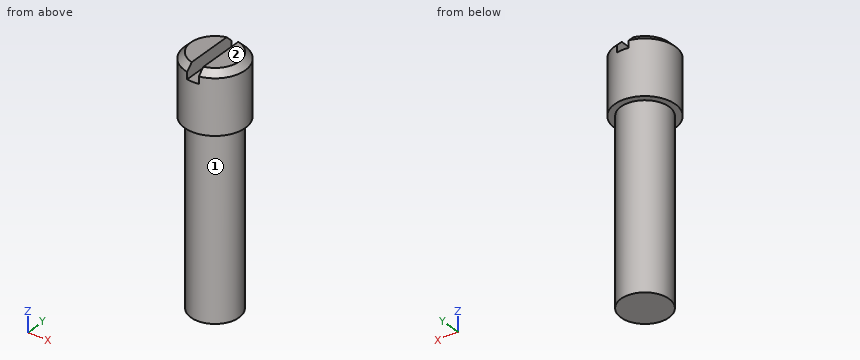
from build123d import *

# Parameters (mm, degrees)
ESQUISSE3_W             = 3
ESQUISSE3_H             = 24
CHANFREIN1_SIZE         = 0.6
ESQUISSE6_R             = 3.5
ENL_V_MAT_EXTRU_1_DEPTH = 25.50510151
ESQUISSE7_OUTSIDE_W     = 13.092
ESQUISSE7_OUTSIDE_H     = 13.092
ESQUISSE7_OUTSIDE_R     = 2.375
ENL_V_MAT_EXTRU_2_DEPTH = 18
ESQUISSE8_W             = 1.15
ESQUISSE8_H             = 7.450711795
ENL_V_MAT_EXTRU_3_DEPTH = 1.3


with BuildPart() as part:
    # Esquisse1 → Base-R_volution (revolve)
    with BuildSketch(Plane(origin=(0, 0, 0), x_dir=(1, 0, 0), z_dir=(0, 1, 0)), mode=Mode.PRIVATE) as base_r_volution_sk:
        with BuildLine():
            Line((0, 0), (3.5, 0))
            Line((3.5, 0), (3.5, 3.6))
            ThreePointArc((3.5, 3.6), (3.382842712, 3.882842712), (3.1, 4))
            Line((3.1, 4), (0, 4))
            Line((0, 4), (0, 0))
        make_face()
    revolve(base_r_volution_sk.sketch.rotate(Axis((0, 0, 0), (0, 0, -1)), 180), axis=Axis((0, 0, 0), (0, 0, -1)))

    # Esquisse3 → Boss.-R_vol.1 (revolve)
    with BuildSketch(Plane(origin=(0, 0, 0), x_dir=(1, 0, 0), z_dir=(0, 1, 0))):
        with Locations((1.5, -12)):
            Rectangle(ESQUISSE3_W, ESQUISSE3_H)
    revolve(axis=Axis((0, 0, 0), (0, 0, 1)))

    # Chanfrein1
    chanfrein1_edges = [part.edges().sort_by_distance(p)[0] for p in [
        (-3, 0, 24),
    ]]
    chamfer(chanfrein1_edges, length=CHANFREIN1_SIZE)

    # Esquisse6 → Enl_v. mat.-Extru.1 (cut, through all)
    with BuildSketch(Plane.XY):
        Circle(ESQUISSE6_R)
    extrude(amount=-ENL_V_MAT_EXTRU_1_DEPTH, mode=Mode.SUBTRACT)

    # Esquisse7 outside → Enl_v. mat.-Extru.2 (cut)
    with BuildSketch(Plane(origin=(0, 0, 0), x_dir=(-1, 0, 0), z_dir=(0, 0, -1))):
        Rectangle(ESQUISSE7_OUTSIDE_W, ESQUISSE7_OUTSIDE_H)
        Circle(ESQUISSE7_OUTSIDE_R, mode=Mode.SUBTRACT)
    extrude(amount=-ENL_V_MAT_EXTRU_2_DEPTH, mode=Mode.SUBTRACT)

    # Esquisse8 → Enl_v. mat.-Extru.3 (cut)
    with BuildSketch(Plane.XY.offset(24)):
        with Locations((0, -0.141041798)):
            Rectangle(ESQUISSE8_W, ESQUISSE8_H)
    extrude(amount=-ENL_V_MAT_EXTRU_3_DEPTH, mode=Mode.SUBTRACT)


solid = part.part
Input: part model. Units: mm. Frame: model coordinates. Face numbers are marked on the shaded views. A direction names the side the tool comes from. Coordinates: 2 decimals unless noted, no trailing zeros. Order: outer loops, then holes, each group sorted by start corner. A loop starts at its lowest first (then second) coordinate and runs counter-clockwise, first axis right, second up. Notation, with made-up numbers: M 73.5,60.5 L 93.5,60.5 A19 ccw 93.5,92.5 Z; hole C -39,38.25 d1. An arc over 180 degrees is marked long. Write item = value, one per line. Start each with the question number.
(1) Section C-C on z = 19.75. Output: boundary loops of the cut face in (x, y), and give its area (3 significant figures).
(2) Line query: line 1 along X through (y, z) = (-0.1, 15.25); line 2 along X through (y, z) = (-0.8, 23) (3 decimals); line 3 along Z through (x, y) = (-1.4, -2.2). Output: solid intervals per line, ascending. Write a range as [from, to].
(3) Section A-A on y = 0. Output: boundary loops of the cut face in (x, z) (3 decimals), and give its area (3 significant figures).
(4) Reachability of the marked faces 1 and 2 from +Z, -Z, +X, -X, +Y, -Y: full face, straight path, thin tool, end or side. Return the list, or none.
(5) First-contact query: P1, Ø2, axis at x = -2.5, z = 14, coming from the -Y side; P2, Ø0.6, axis at x = 0, y = 0.5, coming from the +Z side. Flat tips, straight axial feed; report the tip coordinate or a pass-through.
(6) Section B-B on x = 0. Output: boundary loops of the cut face in (y, z) (3 decimals).
(7) Section D-D on z = 1.5. Output: boundary loops of the cut face in (x, y) (3 decimals).
Result set:
q1.outline = C 0,0 d6
q1.area = 28.3 mm²
q2.line_1 = [-2.37, 2.37]
q2.line_2 = [-2.891, -0.575], [0.575, 2.891]
q2.line_3 = [18, 23.79]
q3.outline = M -3,18 L -2.375,18 L -2.375,0 L 2.375,0 L 2.375,18 L 3,18 L 3,23.4 L 2.4,24 L 0.575,24 L 0.575,22.7 L -0.575,22.7 L -0.575,24 L -2.4,24 L -3,23.4 Z
q3.area = 120 mm²
q4.face_1 = -Z
q4.face_2 = +Z, +X, -X, +Y, -Y
q5.P1 = -1.84
q5.P2 = 22.7
q6.outline = M -3,18 L -2.375,18 L -2.375,0 L 2.375,0 L 2.375,18 L 3,18 L 3,22.7 L -3,22.7 Z
q7.outline = C 0,0 d4.75
